Can you work these out from the model? Positions are in its coordinate system, mm. Face numbers are marked on the shaded views. A direction names the side the tool comes from. Give positions to 0.01 mm unless a question says otherwise; leave off trailing zeros. Order: outer loops, then holes, each group sorted by start corner. A loop starts at its lowest first (then second) coordinate and runs counter-clockwise, first axis right, second up. Notation, with made-up numbers: M 2.5,18.25 L 26.5,18.25 A6 ccw 26.5,26.25 Z; hole C 55,-11 d11. An arc over 180 degrees is marked long. Answer as a JSON object with one key per item and string values.
```python
from build123d import *

# Parameters (mm, degrees)
SKETCH2_W            = 228.6
SKETCH2_H            = 203.2
BOSS_EXTRUDE1_DEPTH  = 3.175
SKETCH3_W            = 228.6
SKETCH3_H            = 3.175
BOSS_EXTRUDE2_DEPTH  = 127
FILLET1_R            = 3.175
FILLET2_R            = 6.35
SKETCH4_R            = 2.54
SKETCH4_R_2          = 2.15
SKETCH4_R_3          = 3.175
CUT_EXTRUDE1_DEPTH   = 265.612965007
CONVERT_SOLID1_START = -114.3
CONVERT_SOLID1_DEPTH = 228.6
SKETCH9_R            = 4.7625
CUT_EXTRUDE2_DEPTH   = 199.7864432


# Read off the part's stored shape, not the designer's step: Convert-Solid1
with BuildPart() as part:
    # Sketch2 → Boss-Extrude1 (new body)
    with BuildSketch(Plane.XY):
        Rectangle(SKETCH2_W, SKETCH2_H)
    extrude(amount=BOSS_EXTRUDE1_DEPTH)

    # Sketch3 → Boss-Extrude2 (add)
    with BuildSketch(Plane.XY.offset(3.175)):
        with Locations((0, -100.0125)):
            Rectangle(SKETCH3_W, SKETCH3_H)
    extrude(amount=BOSS_EXTRUDE2_DEPTH)

    # Fillet1
    fillet1_edges = [part.edges().sort_by_distance(p)[0] for p in [
        (0, -98.425, 3.175),
        (0, -101.6, 0),
    ]]
    fillet(fillet1_edges, radius=FILLET1_R)

    # Fillet2
    fillet2_edges = [part.edges().sort_by_distance(p)[0] for p in [
        (-114.3, -100.0125, 130.175),
        (114.3, -100.0125, 130.175),
        (-114.3, 101.6, 1.5875),
        (114.3, 101.6, 1.5875),
    ]]
    fillet(fillet2_edges, radius=FILLET2_R)

    # Sketch4 → Cut-Extrude1 (cut, through all)
    with BuildSketch(Plane(origin=(0, -98.425, 0), x_dir=(1, 0, 0), z_dir=(0, 1, 0))):
        with Locations(Location((-104.14, -26.035, 0), (0, 0, 270))):
            Circle(SKETCH4_R)
        with Locations(Location((-104.14, -102.4636, 0), (0, 0, 270))):
            Circle(SKETCH4_R)
        with Locations(Location((0.4826, -26.035, 0), (0, 0, 270))):
            Circle(SKETCH4_R)
        with Locations(Location((-27.8257, -102.4636, 0), (0, 0, 270))):
            Circle(SKETCH4_R)
        with Locations(Location((68.25, -79.2493, 0), (0, 0, 270))):
            Circle(SKETCH4_R_2)
        with Locations(Location((97.95, -79.2493, 0), (0, 0, 270))):
            Circle(SKETCH4_R_2)
        with Locations(Location((68.25, -49.2493, 0), (0, 0, 270))):
            Circle(SKETCH4_R_2)
        with Locations(Location((97.95, -49.2493, 0), (0, 0, 270))):
            Circle(SKETCH4_R_2)
        with Locations(Location((-65.9257, -64.2493, 0), (0, 0, 270))):
            Circle(SKETCH4_R_3)
    extrude(amount=-CUT_EXTRUDE1_DEPTH, mode=Mode.SUBTRACT)

    # Convert-Solid1 outline → Convert-Solid1 (cut)
    with BuildSketch(Plane.YZ.offset(CONVERT_SOLID1_START)):
        with BuildLine():
            ThreePointArc((-95.25, 1.5875), (-98.617596045, 2.982403955), (-100.0125, 6.35))
            Line((-100.0125, 6.35), (-100.0125, 130.175))
            Line((-100.0125, 130.175), (-101.6, 130.175))
            Line((-101.6, 130.175), (-101.6, 3.175))
            ThreePointArc((-101.6, 3.175), (-100.67006403, 0.92993597), (-98.425, 0))
            Line((-98.425, 0), (101.6, 0))
            Line((101.6, 0), (101.6, 1.5875))
            Line((101.6, 1.5875), (-95.25, 1.5875))
        make_face()
    extrude(amount=CONVERT_SOLID1_DEPTH, mode=Mode.SUBTRACT)

    # Sketch9 → Cut-Extrude2 (cut, through all)
    with BuildSketch(Plane.XY.offset(3.175)):
        with Locations((-82.55, 82.55)):
            Circle(SKETCH9_R)
        with Locations((82.55, 82.55)):
            Circle(SKETCH9_R)
        with Locations((38.1, -63.5)):
            Circle(SKETCH9_R)
    extrude(amount=-CUT_EXTRUDE2_DEPTH, mode=Mode.SUBTRACT)


solid = part.part
```
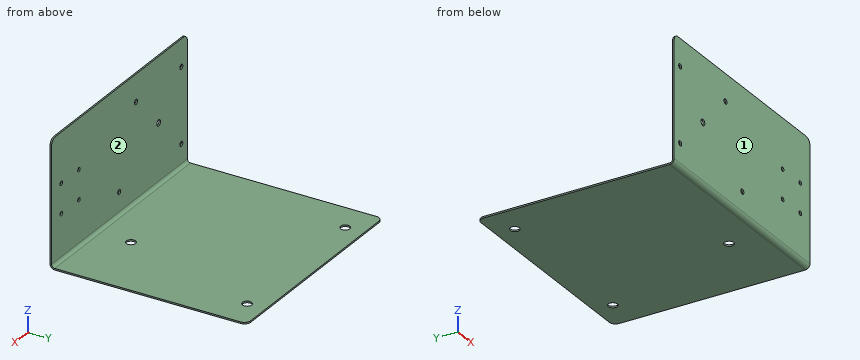
1) I want a section at D-D on z = 117. Write out the boundary of the cut face in (x, y) (1 decimal).
Results found:
{"outline": "M -114.3,-100 L 114.3,-100 L 114.3,-98.4 L -114.3,-98.4 Z"}
2) For the marked faces 1 and 2, which set-ups out of +Z, -Z, +X, -X, +Y, -Y let a thin tool reach every point of the face, with its end or its side?
Results found:
{"face 1": "+Z, -Z, +X, -X, -Y", "face 2": "+Z, +X, -X, +Y"}
3) I'm going to push flat-ended pins straight in: pin 1 Ø8 at (x, y) = (71, 12.5) entering from +Z (3 decimals); pin 2 Ø7 at (x, z) = (68.25, 79.25) entering from +Y (3 decimals). Where does each tip first touch, or does it pass through?
Results found:
{"pin 1": "stops at z = 3.175", "pin 2": "stops at y = -98.425"}
4) I need wall thicknesses on L1, parallel to Z at x = 68, y = -99 (3 decimals); L2, parallel to Z at x = 88.5, y = 59.5 (1 decimal); L3, parallel to Y at x = -66.5, z = 96.5 (1 decimal). Which ranges of each line are inside material? Lowest first, please.
Results found:
{"L1": "z = 3.414 to 47.114, 51.385 to 77.114, 81.385 to 130.175", "L2": "z = 1.6 to 3.2", "L3": "y = -100 to -98.4"}
5) I want a section at B-B on y = -63.5. Write out the boundary of the cut face in (x, z) (1 decimal), and give its area (3 significant figures).
Results found:
{"outline": "M -114.3,1.6 L 33.3,1.6 L 33.3,3.2 L -114.3,3.2 Z; M 42.9,1.6 L 114.3,1.6 L 114.3,3.2 L 42.9,3.2 Z", "area": "348 mm²"}
6) I want a section at C-C on y = 82.55. Write out the boundary of the cut face in (x, z) (1 decimal).
Results found:
{"outline": "M -114.3,1.6 L -87.3,1.6 L -87.3,3.2 L -114.3,3.2 Z; M -77.8,1.6 L 77.8,1.6 L 77.8,3.2 L -77.8,3.2 Z; M 87.3,1.6 L 114.3,1.6 L 114.3,3.2 L 87.3,3.2 Z"}
